from build123d import *

# Parameters (mm, degrees)
SKETCH1_R           = 24
SKETCH1_R_2         = 2.4
BOSS_EXTRUDE1_DEPTH = 2.98
CUT_EXTRUDE1_DEPTH  = 0.8
SKETCH3_R           = 5.5
CUT_EXTRUDE2_DEPTH  = 35.011062906
CHAMFER1_SIZE       = 1
SKETCH4_R           = 12
CUT_EXTRUDE3_DEPTH  = 1


with BuildPart() as part:
    # Sketch1 → Boss-Extrude1 (new body)
    with BuildSketch(Plane(origin=(0, 0, 0), x_dir=(1, 0, 0), z_dir=(0, 1, 0))):
        with Locations(Location((0, 0, 0), (0, 0, 270))):
            Circle(SKETCH1_R)
        with Locations(Location((0, 18, 0), (0, 0, 270))):
            Circle(SKETCH1_R_2, mode=Mode.SUBTRACT)
        with Locations(Location((-18, 0, 0), (0, 0, 270))):
            Circle(SKETCH1_R_2, mode=Mode.SUBTRACT)
        with Locations(Location((0, -18, 0), (0, 0, 270))):
            Circle(SKETCH1_R_2, mode=Mode.SUBTRACT)
        with Locations(Location((18, 0, 0), (0, 0, 270))):
            Circle(SKETCH1_R_2, mode=Mode.SUBTRACT)
    extrude(amount=BOSS_EXTRUDE1_DEPTH)

    # Sketch2 → Cut-Extrude1 (cut)
    with BuildSketch(Plane(origin=(0, 2.98, 0), x_dir=(1, 0, 0), z_dir=(0, 1, 0))):
        with BuildLine():
            Line((4.989999, 2.798442301), (4.989999, -2.798442301))
            Line((4.989999, -2.798442301), (6.819742519, -3.121075451))
            ThreePointArc((6.819742519, -3.121075451), (5.052929001, -5.542373906), (2.479055714, -7.078437876))
            Line((2.479055714, -7.078437876), (2.198435941, -5.663259169))
            ThreePointArc((2.198435941, -5.663259169), (0, -6.075), (-2.198435941, -5.663259169))
            Line((-2.198435941, -5.663259169), (-2.479055714, -7.078437876))
            ThreePointArc((-2.479055714, -7.078437876), (-5.303300859, -5.303300859), (-7.078437876, -2.479055714))
            Line((-7.078437876, -2.479055714), (-5.663259169, -2.198435941))
            ThreePointArc((-5.663259169, -2.198435941), (-6.075, 0), (-5.663259169, 2.198435941))
            Line((-5.663259169, 2.198435941), (-7.078437876, 2.479055714))
            ThreePointArc((-7.078437876, 2.479055714), (-5.303300859, 5.303300859), (-2.479055714, 7.078437876))
            Line((-2.479055714, 7.078437876), (-2.198435941, 5.663259169))
            ThreePointArc((-2.198435941, 5.663259169), (0, 6.075), (2.198435941, 5.663259169))
            Line((2.198435941, 5.663259169), (2.479055714, 7.078437876))
            ThreePointArc((2.479055714, 7.078437876), (5.052929001, 5.542373906), (6.819742519, 3.121075451))
            Line((6.819742519, 3.121075451), (4.989999, 2.798442301))
        make_face()
    extrude(amount=-CUT_EXTRUDE1_DEPTH, mode=Mode.SUBTRACT)

    # Sketch3 → Cut-Extrude2 (cut, through all)
    with BuildSketch(Plane(origin=(0, 2.18, 0), x_dir=(1, 0, 0), z_dir=(0, 1, 0))):
        with Locations(Location((0, 0, 0), (0, 0, 270))):
            Circle(SKETCH3_R)
    extrude(amount=-CUT_EXTRUDE2_DEPTH, mode=Mode.SUBTRACT)

    # Chamfer1
    chamfer1_edges = [part.edges().sort_by_distance(p)[0] for p in [
        (0, 2.98, -20.4),
        (-18, 2.98, -2.4),
        (0, 2.98, 15.6),
        (18, 2.98, -2.4),
    ]]
    chamfer(chamfer1_edges, length=CHAMFER1_SIZE)

    # Sketch4 → Cut-Extrude3 (cut)
    with BuildSketch(Plane.XZ):
        with Locations(Location((0, 0, 0), (0, 0, 270))):
            Circle(SKETCH4_R)
    extrude(amount=-CUT_EXTRUDE3_DEPTH, mode=Mode.SUBTRACT)


solid = part.part
Can you work these out from the model? Positions are in its coordinate system, mm. A direction names the side the tool comes from. Round coordinates to 2 decimals unless told otherwise and drop trailing zeros. Order: outer loops, then holes, each group sorted by start corner. A loop starts at its lowest first (then second) coordinate and runs counter-clockwise, first axis right, second up. Notation, with made-up numbers: M 34,47 L 69,47 A23 cw 69,66 Z; hole C 80,73.5 d6. An arc over 180 degrees is marked long. Use a Markdown table: item, result.
1) Imagine slicing it at C-C (x = 18). List the corners of the cut face in (y, z) for me, then the cut area to 3 significant figures.
Geometry says:
| item | result |
|---|---|
| outline | M 0,-15.87 L 2.98,-15.87 L 2.98,-3.4 L 1.98,-2.4 L 0,-2.4 Z; M 0,2.4 L 1.98,2.4 L 2.98,3.4 L 2.98,15.87 L 0,15.87 Z |
| area | 79.3 mm² |
2) Imagine slicing it at D-D (z = -10.5). List the corners of the cut face in (x, y) for me, then the cut area to 3 significant figures.
Geometry says:
| item | result |
|---|---|
| outline | M -21.58,0 L -5.81,0 L -5.81,1 L 5.81,1 L 5.81,0 L 21.58,0 L 21.58,2.98 L -21.58,2.98 Z |
| area | 117 mm² |
3) If I drill on line 1 along X through (y, z) = (1.3, 0); line 2 along X through (y, z) = (0.3, 0); line 3 along Z through (x, y) = (1, 2.7), over which ranges is the centre line in solid material (lowest first)?
Geometry says:
| item | result |
|---|---|
| line 1 | x = -24 to -20.4, -15.6 to -5.5, 5.5 to 15.6, 20.4 to 24 |
| line 2 | x = -24 to -20.4, -15.6 to -12, 12 to 15.6, 20.4 to 24 |
| line 3 | z = -23.98 to -20.96, -15.04 to -5.99, 5.99 to 15.04, 20.96 to 23.98 |
4) I'm going to push flat-ended pins straight in: P1, Ø1, axis at y = 0.5, z = -15, coming from the +X side; P2, Ø12, axis at x = -1.5, z = 4.5, coming from the -Y side; P3, Ø4.5, axis at x = 18, z = 0, coming from the +Y side; P4, Ø1.5, axis at y = 1.5, z = -18.5, coming from the -X side. Where does each tip first touch, or does it pass through?
Geometry says:
| item | result |
|---|---|
| P1 | stops at x = 19.12 |
| P2 | stops at y = 1 |
| P3 | passes through |
| P4 | stops at x = -16.15 |
5) On a 3-axis mill with a long thin cutter (end or side, diameter ignored), from which of +Z, -Z, +X, -X, +Y, -Y can I reach the whole of each face in a straight line? I mean faces 4 (the face through (3.604, 0.493, -11.446)), 5 (the face through (0.106, 0.976, 15.602)), 6 (the face through (-5.24, 2.18, -2.13)). Say none if no direction works.
Geometry says:
| item | result |
|---|---|
| face 4 | -Y |
| face 5 | +Y, -Y |
| face 6 | +Y |
6) Imagine slicing it at B-B (z = -4). List the corners of the cut face in (x, y) for me.
Geometry says:
| item | result |
|---|---|
| outline | M -23.66,0 L -11.31,0 L -11.31,1 L -3.77,1 L -3.77,2.18 L -6.34,2.18 L -6.34,2.98 L -23.66,2.98 Z; M 3.77,1 L 11.31,1 L 11.31,0 L 23.66,0 L 23.66,2.98 L 6.34,2.98 L 6.34,2.18 L 3.77,2.18 Z |
7) Imagine slicing it at A-A (x = 0). List the corners of the cut face in (y, z) for me (3 decimals).
Geometry says:
| item | result |
|---|---|
| outline | M 0,-24 L 2.98,-24 L 2.98,-21.4 L 1.98,-20.4 L 0,-20.4 Z; M 0,-15.6 L 1.98,-15.6 L 2.98,-14.6 L 2.98,-6.075 L 2.18,-6.075 L 2.18,-5.5 L 1,-5.5 L 1,-12 L 0,-12 Z; M 0,12 L 1,12 L 1,5.5 L 2.18,5.5 L 2.18,6.075 L 2.98,6.075 L 2.98,14.6 L 1.98,15.6 L 0,15.6 Z; M 0,20.4 L 1.98,20.4 L 2.98,21.4 L 2.98,24 L 0,24 Z |
8) If we mould it in two halves opening along X, with no side actions, what happens to faces 1 (the face through (6, 0, -11)), 2 (the face through (-5.27, 2.586, 5.336)), 3 (the face through (7.21, 1.47, 22.89))? For each: +X half, -X half, draft (parallel to the pull), parting line (faces both ways), or undercut.
Geometry says:
| item | result |
|---|---|
| face 1 | draft |
| face 2 | undercut |
| face 3 | parting line |
